Check sheet for the drawn part. Datum: minimum x, y, z corner. Units: mm. A direction names the side the tool comes from. Coordinates: 2 decimals unless noted, no trailing zeros. Loops run counter-clockwise (first coordinate to the right, second up) from the corner with the lowest first, then second, coordinate; pieces in that order, holes last.
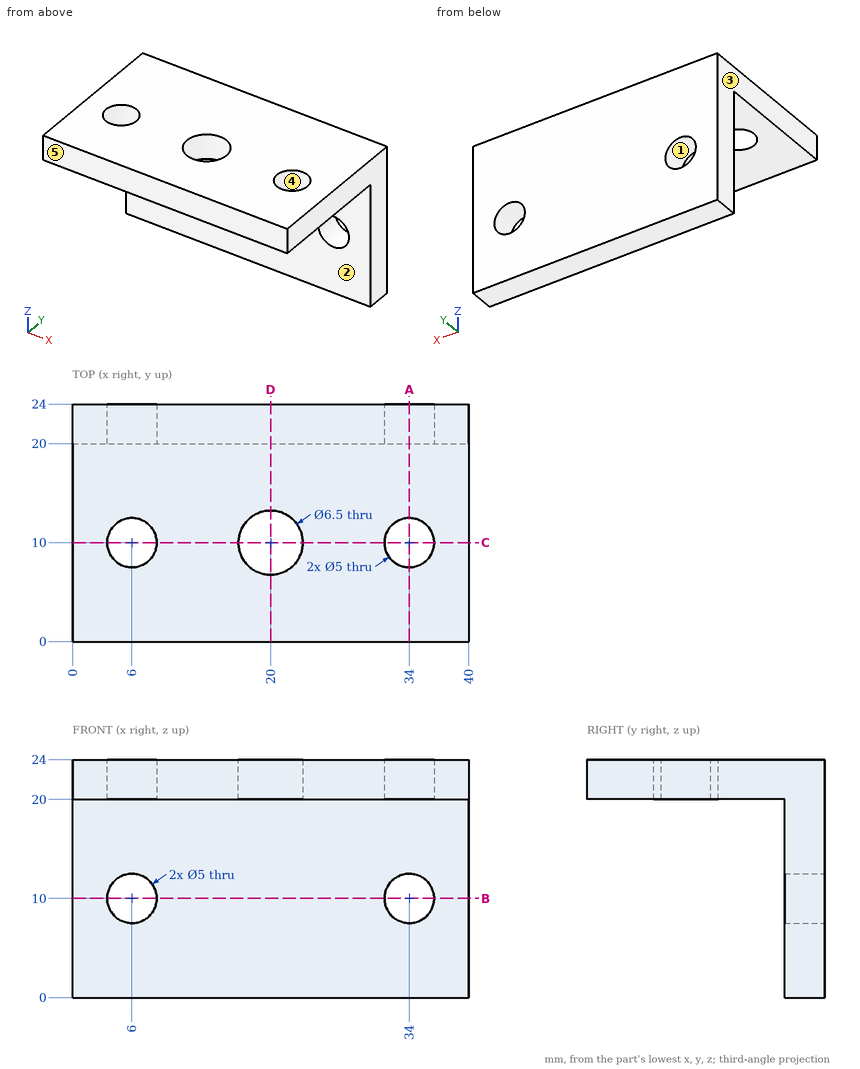
(1) Sectioned sample at C-C on y = 10. Record the cut outline in (x, z).
Findings:
outline: (0, 20) - (3.5, 20) - (3.5, 24) - (0, 24) - close; (8.5, 20) - (16.75, 20) - (16.75, 24) - (8.5, 24) - close; (23.25, 20) - (31.5, 20) - (31.5, 24) - (23.25, 24) - close; (36.5, 20) - (40, 20) - (40, 24) - (36.5, 24) - close
(2) Sectioned sample at D-D on x = 20. Record the cut outline in (y, z), and give its area (3 significant figures).
Findings:
outline: (0, 20) - (6.75, 20) - (6.75, 24) - (0, 24) - close; (13.25, 20) - (20, 20) - (20, 0) - (24, 0) - (24, 24) - (13.25, 24) - close
area: 150 mm2
(3) Draft check along Y on the marked faces 3, 4 and 5. Enter one of: +Y half, -Y half, draft (parallel to the pull), parting line (faces both ways), or undercut.
Findings:
face 3: draft
face 4: undercut
face 5: -Y half
(4) Sectioned sample at A-A on x = 34. Record the cut outline in (y, z), and give its area (3 significant figures).
Findings:
outline: (0, 20) - (7.5, 20) - (7.5, 24) - (0, 24) - close; (12.5, 20) - (20, 20) - (20, 12.5) - (24, 12.5) - (24, 24) - (12.5, 24) - close; (20, 0) - (24, 0) - (24, 7.5) - (20, 7.5) - close
area: 136 mm2
(5) Sectioned sample at B-B on z = 10. Record the cut outline in (x, y), and give its area (3 significant figures).
Findings:
outline: (0, 20) - (3.5, 20) - (3.5, 24) - (0, 24) - close; (8.5, 20) - (31.5, 20) - (31.5, 24) - (8.5, 24) - close; (36.5, 20) - (40, 20) - (40, 24) - (36.5, 24) - close
area: 120 mm2
(6) Access from +Z, -Z, +X, -X, +Y, -Y to the whole of each face (thin tool, end or side, straight path). Record for the marked faces 1 and 2.
Findings:
face 1: +Y, -Y
face 2: -Z, +X, -X, -Y
(7) Gauge pin test, flat ends, axial feed: pin 1 Ø3 at (x, z) = (6, 10) entering from +Y; pin 2 Ø10 at (x, y) = (22.5, 6.5) entering from -Z; pin 3 Ø5 at (x, z) = (7.5, 13) entering from -Y. Record the tip position at first contact, or that the pin passes through.
Findings:
pin 1: passes through
pin 2: stops at z = 20
pin 3: stops at y = 20
(8) Scan lines: L1, parallel to X at y = 21.8, z = 10; L2, parallel to X at y = 10, z = 22.7; L3, parallel to Z at x = 34, y = 22.8. Record each from-to range of solid material in increasing order.
Findings:
L1: x = 0 to 3.5, 8.5 to 31.5, 36.5 to 40
L2: x = 0 to 3.5, 8.5 to 16.75, 23.25 to 31.5, 36.5 to 40
L3: z = 0 to 7.5, 12.5 to 24
